Work out the finished part from the listing and answer in its coordinate system (mm). Face numbers are marked on the shaded views. Round coordinates to 2 decimals unless told otherwise and drop trailing zeros. Write each loop counter-clockwise with the first axis right and the second up, starting at its lowest first coordinate (ties: lowest second). Pieces come first, ordered by that corner, then holes. Notation, with made-up numbers: (-10, -34) - (-4, -34) arc R22 ccw to (-4, -18) - close; hole circle Ø7 at (41.5, 9). An arc over 180 degrees is marked (long way). Answer as a JSON object with one key per item and string values.
```python
from build123d import *

# Parameters (mm, degrees)
SKETCH1_R             = 17.399
BOSS_EXTRUDE1_DEPTH   = 38.1
SKETCH1_R_2           = 29.21
SKETCH1_R_3           = 2.2225
BOSS_EXTRUDE1_2_DEPTH = 38.1
BOSS_EXTRUDE2_DEPTH   = 2.54


with BuildPart() as part:
    # Sketch1 → Boss-Extrude1 (new body)
    with BuildSketch(Plane(origin=(0, 0, 0), x_dir=(1, 0, 0), z_dir=(0, 1, 0))):
        with Locations(Location((0, 0, 0), (0, 0, 90))):
            Circle(SKETCH1_R)
    extrude(amount=BOSS_EXTRUDE1_DEPTH)



with BuildPart() as body_2:
    # Sketch1 → Boss-Extrude1 2 (new body)
    with BuildSketch(Plane(origin=(0, 0, 0), x_dir=(1, 0, 0), z_dir=(0, 1, 0))):
        Polygon((0, -30.48), (30.48, -30.48), (30.48, 30.48), (-30.48, 30.48), (-30.48, -30.48), align=None)
        with Locations(Location((0, 0, 0), (0, 0, 90))):
            Circle(SKETCH1_R_2, mode=Mode.SUBTRACT)
        with Locations(Location((-25.4, 25.4, 0), (0, 0, 90))):
            Circle(SKETCH1_R_3, mode=Mode.SUBTRACT)
        with Locations(Location((-25.4, -25.4, 0), (0, 0, 90))):
            Circle(SKETCH1_R_3, mode=Mode.SUBTRACT)
        with Locations(Location((25.4, -25.4, 0), (0, 0, 90))):
            Circle(SKETCH1_R_3, mode=Mode.SUBTRACT)
        with Locations(Location((25.4, 25.4, 0), (0, 0, 90))):
            Circle(SKETCH1_R_3, mode=Mode.SUBTRACT)
    extrude(amount=BOSS_EXTRUDE1_2_DEPTH)


with BuildPart() as part_1:
    add(part.part)

    add(body_2.part)  # Boss-Extrude2 merges body 2
    # Sketch2 → Boss-Extrude2 (add)
    with BuildSketch(Plane.XZ):
        with BuildLine():
            Line((-10.626679764, 28.595751034), (-6.570086281, 16.110840054))
            ThreePointArc((-6.570086281, 16.110840054), (-5.376586685, 16.547432327), (-4.15440273, 16.89574322))
            Line((-4.15440273, 16.89574322), (-8.210996213, 29.3806542))
            Line((-8.210996213, 29.3806542), (-10.626679764, 28.595751034))
        make_face()
        with BuildLine():
            Line((23.912350718, 18.943146073), (13.292051101, 11.227046741))
            ThreePointArc((13.292051101, 11.227046741), (14.076086685, 10.226875605), (14.785025642, 9.172143575))
            Line((14.785025642, 9.172143575), (25.405325259, 16.888242907))
            Line((25.405325259, 16.888242907), (23.912350718, 18.943146073))
        make_face()
        with BuildLine():
            ThreePointArc((14.785025642, -9.172143575), (14.076086685, -10.226875605), (13.292051101, -11.227046741))
            Line((13.292051101, -11.227046741), (23.912350718, -18.943146073))
            Line((23.912350718, -18.943146073), (25.405325259, -16.888242907))
            Line((25.405325259, -16.888242907), (14.785025642, -9.172143575))
        make_face()
        with BuildLine():
            ThreePointArc((-4.15440273, -16.89574322), (-5.376586685, -16.547432327), (-6.570086281, -16.110840054))
            Line((-6.570086281, -16.110840054), (-10.626679764, -28.595751034))
            Line((-10.626679764, -28.595751034), (-8.210996213, -29.3806542))
            Line((-8.210996213, -29.3806542), (-4.15440273, -16.89574322))
        make_face()
        with BuildLine():
            ThreePointArc((-17.352587732, -1.27), (-17.387393062, -0.635423894), (-17.399, 0))
            Line((-17.399, 0), (-30.48, 0))
            Line((-30.48, 0), (-30.48, -1.27))
            Line((-30.48, -1.27), (-17.352587732, -1.27))
        make_face()
        with BuildLine():
            Line((-30.48, 0), (-17.399, 0))
            ThreePointArc((-17.399, 0), (-17.387393062, 0.635423894), (-17.352587732, 1.27))
            Line((-17.352587732, 1.27), (-30.48, 1.27))
            Line((-30.48, 1.27), (-30.48, 0))
        make_face()
    extrude(amount=-BOSS_EXTRUDE2_DEPTH)


solid = part_1.part
```
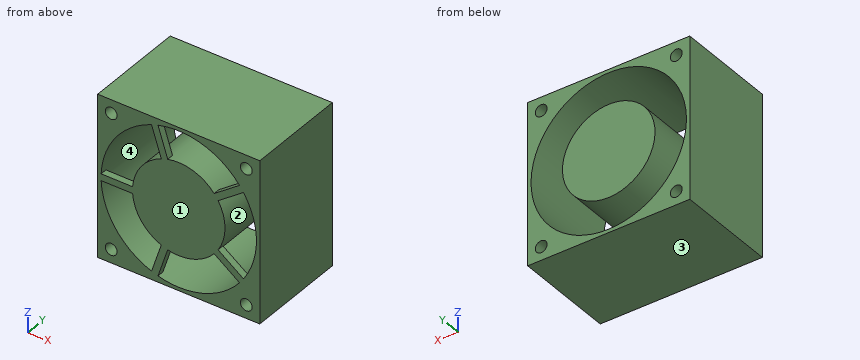
Item 1: Consider line 1 along X through (y, z) = (19, 0); line 2 along Z through (x, y) = (-25.4, 20); line 3 along Z through (x, y) = (15.5, 3). Determine where each line is inside the solid, lowest interval first.
Results found:
{"line 1": "-30.48 to -29.21, -17.4 to 17.4, 29.21 to 30.48", "line 2": "-30.48 to -27.62, -23.18 to -14.42, 14.42 to 23.18, 27.62 to 30.48", "line 3": "-30.48 to -24.76, -7.9 to 7.9, 24.76 to 30.48"}
Item 2: A cutting plane is placed at C-C (z = -10). Write down the section's boundary in (x, y), and give its area (3 significant figures).
Results found:
{"outline": "(-30.48, 0) - (-27.44, 0) - (-27.44, 38.1) - (-30.48, 38.1) - close; (-14.24, 0) - (15.92, 0) - (15.92, 2.54) - (14.24, 2.54) - (14.24, 38.1) - (-14.24, 38.1) - close; (27.44, 0) - (30.48, 0) - (30.48, 38.1) - (27.44, 38.1) - close", "area": "1,320 mm²"}
Item 3: A cutting plane is placed at D-D (z = 25.4). Write down the section's boundary in (x, y).
Results found:
{"outline": "(-30.48, 0) - (-27.62, 0) - (-27.62, 38.1) - (-30.48, 38.1) - close; (-23.18, 0) - (-14.42, 0) - (-14.42, 38.1) - (-23.18, 38.1) - close; (-9.59, 0) - (-6.92, 0) - (-6.92, 2.54) - (-9.59, 2.54) - close; (14.42, 0) - (23.18, 0) - (23.18, 38.1) - (14.42, 38.1) - close; (27.62, 0) - (30.48, 0) - (30.48, 38.1) - (27.62, 38.1) - close"}
Item 4: A cutting plane is placed at B-B (x = 0). Write down the section's boundary in (y, z), and give its area (3 significant figures).
Results found:
{"outline": "(0, -30.48) - (38.1, -30.48) - (38.1, -29.21) - (0, -29.21) - close; (0, -17.4) - (38.1, -17.4) - (38.1, 17.4) - (0, 17.4) - close; (0, 29.21) - (38.1, 29.21) - (38.1, 30.48) - (0, 30.48) - close", "area": "1,420 mm²"}
Item 5: Each of these flat-tipped pins is pushed along its axis until it touches: P1, Ø3.5, axis at x = 25.4, z = 25.4, coming from the +Y side; P2, Ø5, axis at x = -7.5, z = -19.5, coming from the +Y side. Where does it stop, or does it pass through?
Results found:
{"P1": "through", "P2": "y = 2.54"}
Item 6: Determine the mould class of the marked faces 1, 2, 3 and 4 for opening direction Z: pulls with the +Z half, pulls with the -Z half, needs draft (parallel to the pull), parting line crosses it, or undercut.
Results found:
{"face 1": "needs draft", "face 2": "undercut", "face 3": "pulls with the -Z half", "face 4": "undercut"}
Item 7: A cutting plane is placed at A-A (y = 22). Write down the section's boundary in (x, z) (1 decimal).
Results found:
{"outline": "(-30.5, -30.5) - (30.5, -30.5) - (30.5, 30.5) - (-30.5, 30.5) - close; circle Ø34.8 at (0, 0); hole circle Ø58.4 at (0, 0); hole circle Ø4.4 at (-25.4, -25.4); hole circle Ø4.4 at (-25.4, 25.4); hole circle Ø4.4 at (25.4, -25.4); hole circle Ø4.4 at (25.4, 25.4)"}
